For this review, take the finished solid that the model builds, in its own axes (mm). Face numbers are marked on the shaded views. A direction names the side the tool comes from. Coordinates: 2 decimals unless noted, no trailing zeros. Loops run counter-clockwise (first coordinate to the right, second up) from the corner with the lowest first, then second, coordinate; pieces in that order, holes last. Notation, with made-up numbers: (45, 20.5) - (79, 20.5) arc R21 cw to (79, 28.5) - close; hole circle Ø4 at (0.5, 69). An arc over 180 degrees is marked (long way). One line per item, written item: value. Start each with the question number.
1. Take a section at C-C, the plane y = -71.25. State the section outline as (x, z) points, and give its area (3 significant figures).
2. Take a section at B-B, the plane x = -43.75. State the section outline as (y, z) points.
3. Take a section at D-D, the plane x = -47.25. State the section outline as (y, z) points.
4. For the marked faces 1 and 2, list the 3-axis set-ups (+Z, -Z, +X, -X, +Y, -Y) from which the entire face can be reached by the end or side of a thin tool; tool diameter is ignored.
5. To check wall thickness, follow line 1 (X direction, y = -72.25, z = 2.7); line 2 (Z direction, x = -46.5, y = -67); line 3 (Y direction, x = -42.5, z = 2.3). State the ranges of each line that lie inside material, in increasing order. Write a range as from..to.
6. Insertion check: pin 1 (4 mm diameter, centred on x = -46.73, y = -71.86, fed in from +Z); pin 2 (3 mm diameter, centred on x = -37.5, y = -66.5, fed in from -Z); pin 3 (1 mm diameter, centred on x = -48.5, z = 3, fed in from +Y). Each pin has a flat end and moves straight along its axis. Give the tip position at first contact, or say it passes through.
7. The part is to be moulded in two halves that separate along Y. For the marked faces 3, 4 and 5, say which applies: released by +Y, released by -Y, zero draft, split by the parting line, or undercut.
8. Take a section at A-A, the plane y = -66. State the section outline as (x, z) points.
```python
from build123d import *

# Parameters (mm, degrees)
SKETCH1_R           = 8
SKETCH1_R_2         = 6
SKETCH1_R_3         = 1.25
SKETCH1_R_4         = 1.5
BOSS_EXTRUDE1_DEPTH = 3.5
SKETCH2_R           = 1.5
BOSS_EXTRUDE2_DEPTH = 2


with BuildPart() as part:
    # Sketch1 → Boss-Extrude1 (new body)
    with BuildSketch(Plane.XY):
        with Locations((-43.483141232, -69.989052064)):
            Circle(SKETCH1_R)
        with Locations((-43.483141232, -69.989052064)):
            Circle(SKETCH1_R_2, mode=Mode.SUBTRACT)
        with Locations((-43.483141232, -69.989052064)):
            Circle(SKETCH1_R)
        with Locations((-40.235545968, -71.864052064)):
            Circle(SKETCH1_R_3, mode=Mode.SUBTRACT)
        with Locations((-46.730736496, -71.864052064)):
            Circle(SKETCH1_R_3, mode=Mode.SUBTRACT)
        with Locations((-43.483141232, -66.239052064)):
            Circle(SKETCH1_R_3, mode=Mode.SUBTRACT)
        with Locations((-43.483141232, -69.989052064)):
            Circle(SKETCH1_R_4, mode=Mode.SUBTRACT)
        with Locations((-43.483141232, -69.989052064)):
            Circle(SKETCH1_R_4)
    extrude(amount=BOSS_EXTRUDE1_DEPTH)

    # Sketch2 → Boss-Extrude2 (add)
    with BuildSketch(Plane(origin=(0, 0, 0), x_dir=(-1, 0, 0), z_dir=(0, 0, -1))):
        with Locations((43.483141232, -69.989052064)):
            Circle(SKETCH2_R)
    extrude(amount=BOSS_EXTRUDE2_DEPTH)


solid = part.part
```
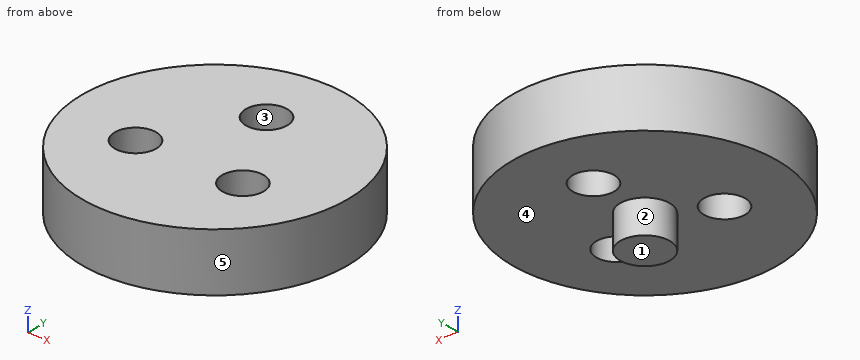
Solutions:
1. outline: (-51.38, 0) - (-47.82, 0) - (-47.82, 3.5) - (-51.38, 3.5) - close; (-45.64, 0) - (-44.3, 0) - (-44.3, -2) - (-42.67, -2) - (-42.67, 0) - (-41.32, 0) - (-41.32, 3.5) - (-45.64, 3.5) - close; (-39.15, 0) - (-35.58, 0) - (-35.58, 3.5) - (-39.15, 3.5) - close
1. area: 43.3 mm2
2. outline: (-77.98, 0) - (-71.47, 0) - (-71.47, -2) - (-68.51, -2) - (-68.51, 0) - (-67.46, 0) - (-67.46, 3.5) - (-77.98, 3.5) - close; (-65.02, 0) - (-61.99, 0) - (-61.99, 3.5) - (-65.02, 3.5) - close
3. outline: (-77.05, 0) - (-73, 0) - (-73, 3.5) - (-77.05, 3.5) - close; (-70.73, 0) - (-62.93, 0) - (-62.93, 3.5) - (-70.73, 3.5) - close
4. face 1: -Z, +X, -X, +Y, -Y
4. face 2: -Z
5. line 1: -51.16..-47.92, -45.54..-41.42, -39.05..-35.81
5. line 2: 0..3.5
5. line 3: -77.93..-67.01, -65.47..-62.05
6. pin 1: z = 3.5
6. pin 2: z = 0
6. pin 3: y = -63.39
7. face 3: undercut
7. face 4: zero draft
7. face 5: split by the parting line
8. outline: (-50.42, 0) - (-44.71, 0) - (-44.71, 3.5) - (-50.42, 3.5) - close; (-42.26, 0) - (-36.55, 0) - (-36.55, 3.5) - (-42.26, 3.5) - close
